Part model, mm, in its own coordinate system. Face numbers are marked on the shaded views. A direction names the side the tool comes from. Coordinates: 2 decimals unless noted, no trailing zeros. Loops run counter-clockwise (first coordinate to the right, second up) from the corner with the lowest first, then second, coordinate; pieces in that order, holes last.
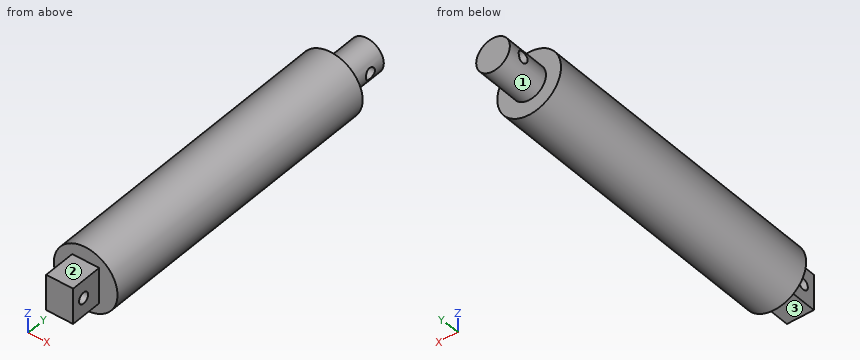
Autodesk Inventor part; units mm, degrees
ref_plane "YZ Plane" through (0, 0, 0) normal (1, 0, 0) x (0, 1, 0)
ref_plane "XZ Plane" through (0, 0, 0) normal (0, 1, 0) x (-1, 0, 0)
ref_plane "XY Plane" through (0, 0, 0) normal (0, 0, 1) x (1, 0, 0)
sketch "Sketch1" plane through (0, 0, 0) normal (0, 1, 0) x (-1, 0, 0)
  circle A0 centre (0, 0) radius 18.034
  dimension "d0" = 36.068
extrude "Extrusion1" add sketch "Sketch1" along normal blind 172.212
sketch "Sketch2" plane through (0, 172.212, 0) normal (0, 1, 0) x (1, 0, 0)
  circle A0 centre (0, 0) radius 9.525
  dimension "d3" = 19.05
extrude "Extrusion2" add sketch "Sketch2" along normal blind 25.4
sketch "Sketch3" plane through (0, 0, 0) normal (0, -1, 0) x (1, 0, 0)
  line L0 (-7.62, -10.16) -> (7.62, -10.16)
  line L1 (7.62, -10.16) -> (7.62, 10.16)
  line L2 (7.62, 10.16) -> (-7.62, 10.16)
  line L3 (-7.62, 10.16) -> (-7.62, -10.16)
  line L4 (-7.62, -10.16) -> (7.62, 10.16) construction
  line L5 (7.62, -10.16) -> (-7.62, 10.16) construction
  point P0 (0, 0)
  dimension "d6" = 15.24
  dimension "d7" = 20.32
extrude "Extrusion3" add sketch "Sketch3" along normal blind 18.288
sketch "Sketch4" plane through (7.62, 0, 10.16) normal (1, 0, 0) x (0, 0, -1)
  line L0 (0, 0) -> (20.32, 0)
  line L1 (20.32, 0) -> (20.32, -18.288)
  point P0 (10.16, 0)
  point P1 (10.16, -10.922)
  dimension "d10" = 10.922
  dimension "d11" = 10.16
hole "Hole1" at (7.62, -10.922, 0) direction (-1, 0, 0) diameter 6.35 end through all
sketch "Sketch5" plane through (7.62, 0, 10.16) normal (1, 0, 0) x (0, 0, -1)
  circle A0 centre (10.16, 188.214) radius 3.175
  line L0 (19.685, 197.612) -> (0.635, 197.612)
  point P0 (10.16, 0)
  dimension "d19" = 6.35
  dimension "d24" = 9.398
extrude "Extrusion4" cut sketch "Sketch5" along normal mid plane 127
properties part number "7.5 inch Linear Actuator"
Q1. Drop flat-ended pins along their axis: P1, Ø4, axis at x = -9, y = 137, coming from the +Z side; P2, Ø5.5, axis at y = -13.5, z = -4, coming from the -X side; P3, Ø7.5, axis at x = -3.5, y = -5.5, coming from the -Z side; P4, Ø12, axis at x = 2, z = 9.5, coming from the +Y side. Give the stop position or say it passes through.
Q2. Saw through at C-C (y = 118.5). List the corners of the cut face in (x, z), plus the area to 3 significant figures.
Q3. Saw through at A-A (z = 0). List the corners of the cut face in (x, y) (3 decimals), plus the area to 3 significant figures.
Q4. Saw through at D-D (z = 12.5). List the corners of the cut face in (x, y).
Q5. Saw through at B-B (x = -1). List the corners of the cut face in (y, z) (3 decimals), plus the area to 3 significant figures.
Q6. Tool access for the marked faces 1, 2 and 3: list every direction of +Z, -Z, +X, -X, +Y, -Y with a clear straight run to the whole face (end or side of a thin tool).
Q7. Probe line 1 (Y direction, x = -1.5, z = 0); line 2 (Y direction, x = 1, z = 2); line 3 (Z direction, x = -0.5, y = 45). List the from-to ranges inside material, lowest first.
Checked values:
1. P1: stops at z = 16.62
1. P2: stops at x = -7.62
1. P3: stops at z = -10.16
1. P4: stops at y = 197.61
2. outline: circle Ø36.07 at (0, 0)
2. area: 1,020 mm2
3. outline: (-18.034, 0) - (-7.62, 0) - (-7.62, -7.747) - (7.62, -7.747) - (7.62, 0) - (18.034, 0) - (18.034, 172.212) - (9.525, 172.212) - (9.525, 185.039) - (-9.525, 185.039) - (-9.525, 172.212) - (-18.034, 172.212) - close; (-9.525, 191.389) - (9.525, 191.389) - (9.525, 197.612) - (-9.525, 197.612) - close; (-7.62, -18.288) - (7.62, -18.288) - (7.62, -14.097) - (-7.62, -14.097) - close
3. area: 6,760 mm2
4. outline: (-13, 0) - (13, 0) - (13, 172.21) - (-13, 172.21) - close
5. outline: (-18.288, -10.16) - (0, -10.16) - (0, -18.006) - (172.212, -18.006) - (172.212, -9.472) - (197.612, -9.472) - (197.612, 9.472) - (172.212, 9.472) - (172.212, 18.006) - (0, 18.006) - (0, 10.16) - (-18.288, 10.16) - close; hole circle Ø6.35 at (-10.922, 0); hole circle Ø6.35 at (188.214, 0)
5. area: 6,990 mm2
6. face 1: +Y
6. face 2: +Z, +X, -X, -Y
6. face 3: -Z, +X, -X, -Y
7. line 1: y = -18.29 to -14.1, -7.75 to 185.04, 191.39 to 197.61
7. line 2: y = -18.29 to -13.39, -8.46 to 185.75, 190.68 to 197.61
7. line 3: z = -18.03 to 18.03
